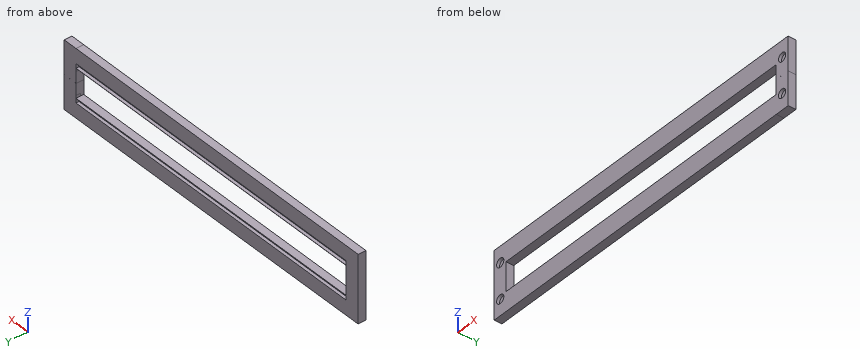
from build123d import *

# Parameters (mm, degrees)
BOSS_EXTRUDE1_DEPTH = 10.16
CUT_EXTRUDE1_DEPTH  = 469.9
SKETCH7_W           = 12.402912868
SKETCH7_H           = 5.692085864
BOSS_EXTRUDE2_DEPTH = 19.05
SKETCH8_W           = 44.473666897
SKETCH8_H           = 10.16
BOSS_EXTRUDE3_DEPTH = 19.05
SKETCH11_R          = 5.7912
CUT_EXTRUDE2_DEPTH  = 3.81


with BuildPart() as part:
    # Sketch1 → Boss-Extrude1 (new body)
    with BuildSketch(Plane(origin=(0, 0, 0), x_dir=(1, 0, 0), z_dir=(0, 1, 0))):
        Polygon((16.038025544, 57.472460937), (-434.826171875, 57.472460937), (-434.826171875, 13.022460937), (-415.790369294, 13.022460937), (-415.790369294, 32.072460937), (16.038025544, 32.072460938), align=None)
        Polygon((35.073828125, 57.472460938), (16.038025544, 57.472460937), (16.038025544, 32.072460938), (16.038025544, 13.022460938), (35.073828125, 13.022460938), align=None)
    extrude(amount=BOSS_EXTRUDE1_DEPTH)

    # Sketch3 → Cut-Extrude1 (cut)
    with BuildSketch(Plane(origin=(35.073828125, 0, 0), x_dir=(0, 0, -1), z_dir=(1, 0, 0))):
        Polygon((38.155998325, 6.152693314), (38.155998325, 10.16), (32.33892355, 10.16), (32.33892355, 6.152693314), (35.247460938, 7.831938158), align=None)
    extrude(amount=-CUT_EXTRUDE1_DEPTH, mode=Mode.SUBTRACT)

    # Sketch7 → Boss-Extrude2 (add)
    with BuildSketch(Plane(origin=(35.073828125, 0, 0), x_dir=(0, 0, -1), z_dir=(1, 0, 0))):
        with Locations((34.557393907, 7.313957068)):
            Rectangle(SKETCH7_W, SKETCH7_H)
    extrude(amount=-BOSS_EXTRUDE2_DEPTH)

    # Sketch8 → Boss-Extrude3 (add)
    with BuildSketch(Plane.ZY.offset(434.826171875)):
        with Locations((-35.23562749, 5.08)):
            Rectangle(SKETCH8_W, SKETCH8_H)
    extrude(amount=-BOSS_EXTRUDE3_DEPTH)

    # Mirror1: part across plane


with BuildPart() as part_1:
    add(part.part)
    add(part.part.mirror(Plane(origin=(-415.776171875, 10.16, -12.998794041), x_dir=(1, 0, 0), z_dir=(0, 0, 1))))

    # Sketch11 → Cut-Extrude2 (cut)
    with BuildSketch(Plane.XZ):
        with Locations((-425.156251148, 10.226790326)):
            Circle(SKETCH11_R)
        with Locations((25.403907398, -36.248045304)):
            Circle(SKETCH11_R)
        with Locations((25.403907398, 10.226790326)):
            Circle(SKETCH11_R)
        with Locations((-425.156251148, -36.248045304)):
            Circle(SKETCH11_R)
    extrude(amount=-CUT_EXTRUDE2_DEPTH, mode=Mode.SUBTRACT)


solid = part_1.part
Model file for the job. Use its own axes, mm. Give positions to 0.01 mm unless a question says otherwise; leave off trailing zeros. Loops run counter-clockwise (first coordinate to the right, second up) from the corner with the lowest first, then second, coordinate; pieces in that order, holes last. Notation, with made-up numbers: (51.5, 78.25) - (55.5, 78.25) arc R12 ccw to (55.5, 90.25) - close; hole circle Ø8 at (40.5, 42.25). An arc over 180 degrees is marked (long way). Use one line per item in the form item = value.
(1) Drop flat-ended pins along their axis: P1, Ø3.5, axis at x = 25.5, z = -36, coming from the -Y side; P2, Ø1, axis at x = -229.5, z = -34.5, coming from the +Y side. Give the stop position or say it passes through.
Determined:
P1 = 3.81
P2 = 7.69
(2) Cut at A-A (x = -205). Give the cut face in (y, z), then the cut area to 3 significant figures.
Determined:
outline = (0, -57.47) - (10.16, -57.47) - (10.16, -38.16) - (6.15, -38.16) - (7.83, -35.25) - (6.15, -32.34) - (10.16, -32.34) - (10.16, -32.07) - (0, -32.07) - close; (0, 6.07) - (10.16, 6.07) - (10.16, 6.34) - (6.15, 6.34) - (7.83, 9.25) - (6.15, 12.16) - (10.16, 12.16) - (10.16, 31.47) - (0, 31.47) - close
area = 479 mm^2
(3) Drill centre lines: L1, parallel to Z at x = -384.5, y = 8; L2, parallel to X at y = 4.25, z = 3; L3, parallel to Z at x = -6.5, y = 3.25. Where is each one in solid material? Low to high.
Determined:
L1 = -57.47 to -38.16, -32.34 to -32.07, 6.07 to 6.34, 12.16 to 31.47
L2 = -434.83 to -415.78, 16.04 to 35.07
L3 = -57.47 to -32.07, 6.07 to 31.47
(4) Cut at B-B (y = 2). Give the cut face in (x, z), then the cut area to 3 significant figures.
Determined:
outline = (-434.83, -57.47) - (35.07, -57.47) - (35.07, -13.02) - (16.04, -13.02) - (16.04, -32.07) - (-415.78, -32.07) - (-415.78, 6.07) - (16.04, 6.07) - (16.04, -12.98) - (35.07, -12.98) - (35.07, 31.47) - (-434.83, 31.47) - close; hole circle Ø11.58 at (-425.16, -36.25); hole circle Ø11.58 at (-425.16, 10.23); hole circle Ø11.58 at (25.4, -36.25); hole circle Ø11.58 at (25.4, 10.23)
area = 24,900 mm^2
